Part model, mm, in its own coordinate system. A direction names the side the tool comes from. Round coordinates to 2 decimals unless told otherwise and drop trailing zeros. Write each loop counter-clockwise with the first axis right and the second up, starting at its lowest first coordinate (ties: lowest second). Pieces come first, ordered by that corner, then holes. Notation, with made-up numbers: M -23.75,7 L 4.25,7 A11 cw 4.25,23 Z; hole C 22.25,76 d11. An arc over 180 degrees is marked long. One line per question, with ' | ' between items. Start each with the question number.
1) Saw through at C-C (x = -7.75). List the corners of the cut face in (y, z).
2) Saw through at B-B (z = -2.2). List the corners of the cut face in (x, y), plus the area to 3 significant figures.
3) Drop flat-ended pins along their axis: pin 1 Ø10 at (x, y) = (3, -2) entering from +Z; pin 2 Ø0.6 at (y, z) = (-3.5, -1.5) entering from +X; pin 3 Ø0.9 at (y, z) = (-7, 1.5) entering from -X; pin 4 Ø0.9 at (x, y) = (-1.5, -2.5) entering from +Z. Give the stop position or say it passes through.
4) Wall check: probe 1 along Z at (x, y) = (-6.75, 7.75); probe 2 along Z at (x, y) = (-6.5, -8.5); probe 3 along Y at (x, z) = (-6.75, 0.55). Give the ranges that are in metal, low to high. Write a range as [from, to].
5) Saw through at A-A (x = -4). List the corners of the cut face in (y, z), plus the area to 3 significant figures.
6) Tool access for faces 4 (the face through (-4, -5, -1.67)), 5 (the face through (-1.3, -4.9, -0.87)), 6 (the face through (-11.5, 5, 1.67)), 7 (the face through (-11.5, -4.9, 1.67)): list every direction of +Z, -Z, +X, -X, +Y, -Y with a clear straight run to the whole face (end or side of a thin tool).
7) Mould opens along Z. For faces 1 (the face through (0, 8.5, 0)), 2 (the face through (-6.4, -4.9, 1.67)), 3 (the face through (-9, 5, -0.87)) say: pulls with the +Z half, pulls with the -Z half, needs draft (parallel to the pull), parting line crosses it, or undercut.
```python
from build123d import *

# Parameters (mm, degrees)
SKIZZE1_W                       = 26
SKIZZE1_H                       = 5
AUFSATZ_LINEAR_AUSTRAGEN1_DEPTH = 8.5
SKIZZE2_W                       = 0.8
SKIZZE2_H                       = 0.8
AUFSATZ_LINEAR_AUSTRAGEN2_DEPTH = 10
SKIZZE3_W                       = 0.8
SKIZZE3_H                       = 0.8
SCHNITT_LINEAR_AUSTRAGEN1_DEPTH = 7
LINEARES_MUSTER1_COUNT          = 10
LINEARES_MUSTER1_PITCH          = 2.54
LINEARES_MUSTER1_COUNT_DIR2     = 2
LINEARES_MUSTER1_PITCH_DIR2     = 2.54


with BuildPart() as part:
    # Skizze1 → Aufsatz-Linear austragen1 (new body)
    with BuildSketch(Plane(origin=(0, 0, 0), x_dir=(1, 0, 0), z_dir=(0, 1, 0))):
        Rectangle(SKIZZE1_W, SKIZZE1_H)
    extrude(amount=AUFSATZ_LINEAR_AUSTRAGEN1_DEPTH)

    # Skizze2 → Aufsatz-Linear austragen2 (add)
    with BuildSketch(Plane(origin=(0, 0, 0), x_dir=(1, 0, 0), z_dir=(0, 1, 0))):
        with Locations((-11.48, -1.27)):
            Rectangle(SKIZZE2_W, SKIZZE2_H)
    aufsatz_linear_austragen2 = extrude(amount=-AUFSATZ_LINEAR_AUSTRAGEN2_DEPTH)

    # Skizze3 → Schnitt-Linear austragen1 (cut)
    with BuildSketch(Plane(origin=(0, 8.5, 0), x_dir=(1, 0, 0), z_dir=(0, 1, 0))):
        with Locations((-11.48, -1.27)):
            Rectangle(SKIZZE3_W, SKIZZE3_H)
    schnitt_linear_austragen1 = extrude(amount=-SCHNITT_LINEAR_AUSTRAGEN1_DEPTH, mode=Mode.SUBTRACT)

    # Lineares Muster1: Aufsatz-Linear austragen2, Schnitt-Linear austragen1 10 × 2
    with Locations(*[(i * LINEARES_MUSTER1_PITCH, 0, -j * LINEARES_MUSTER1_PITCH_DIR2) for i in range(LINEARES_MUSTER1_COUNT) for j in range(LINEARES_MUSTER1_COUNT_DIR2) if (i, j) != (0, 0)]):
        add(aufsatz_linear_austragen2)
        add(schnitt_linear_austragen1, mode=Mode.SUBTRACT)


solid = part.part
```
Answer key:
1) outline: M 0,-2.5 L 8.5,-2.5 L 8.5,2.5 L 0,2.5 Z
2) outline: M -13,0 L 13,0 L 13,8.5 L -13,8.5 Z | area: 221 mm2
3) pin 1: stops at z = 2.5 | pin 2: stops at x = 11.78 | pin 3: stops at x = -11.88 | pin 4: stops at z = 1.67
4) probe 1: z = [-2.5, -1.67], [-0.87, 0.87], [1.67, 2.5] | probe 2: z = [-1.67, -0.87], [0.87, 1.67] | probe 3: y = [0, 8.5]
5) outline: M -10,-1.67 L 0,-1.67 L 0,-2.5 L 8.5,-2.5 L 8.5,-1.67 L 1.5,-1.67 L 1.5,-0.87 L 8.5,-0.87 L 8.5,0.87 L 1.5,0.87 L 1.5,1.67 L 8.5,1.67 L 8.5,2.5 L 0,2.5 L 0,1.67 L -10,1.67 L -10,0.87 L 0,0.87 L 0,-0.87 L -10,-0.87 Z | area: 47.3 mm2
6) face 4: -Z, +X, -X, -Y | face 5: +X, -X, -Y | face 6: +Y | face 7: +Z, +X, -X, -Y
7) face 1: needs draft | face 2: pulls with the +Z half | face 3: undercut
